Design review of the part built by this model. Coordinates are the model's own, in mm. Face numbers are marked on the shaded views. A direction names the side the tool comes from. Coordinates: 2 decimals unless noted, no trailing zeros. Loops run counter-clockwise (first coordinate to the right, second up) from the corner with the lowest first, then second, coordinate; pieces in that order, holes last. Notation, with made-up numbers: (-18, 49) - (24, 49) arc R12 cw to (24, 72) - close; hole circle Ø7 at (25.5, -40). An arc over 180 degrees is marked (long way). Use one line per item in the form item = value. Start each with the question number.
(1) Tool access review of the marked faces 1 and 2: name each direction out of +Z, -Z, +X, -X, +Y, -Y from which nothing blocks a thin tool from reaching the whole face with its end or side.
(2) Add section C-C (z = 3.95). State the section outline as (x, y) points.
(3) Add section D-D (z = 0.6). State the section outline as (x, y) points.
(4) Add section A-A (y = 0). State the section outline as (x, z) points.
(5) For L1, parallel to Z at x = -0.25, y = -7.5; L2, parallel to Y at x = -0.25, z = 1.65; L3, parallel to Z at x = -4.5, y = 1, list the stretches that pass through material, from the lowest coordinate up.
(6) Clearance check with a flat-ended pin moving along its axis: pin 1 Ø1 at (y, z) = (5, 1) entering from -X. State where the tip first meets the part, or that it passes through.
```python
from build123d import *

# Parameters (mm, degrees)
F0_R     = 11.5
F0_R_2   = 6.5
F1_DEPTH = 1.5
F0_R_3   = 4
F2_DEPTH = 2.5
F3_DEPTH = 5.5
F4_SIZE  = 1


with BuildPart() as f1:
    # F0 (on Top) → F1 (new body)
    with BuildSketch(Plane.XY):
        Circle(F0_R)
        Circle(F0_R_2, mode=Mode.SUBTRACT)
    extrude(amount=F1_DEPTH)

    # F0 (on Top) → F2 (join)
    with BuildSketch(Plane.XY):
        Circle(F0_R_2)
        Circle(F0_R_3, mode=Mode.SUBTRACT)
    extrude(amount=F2_DEPTH)

    # F0 (on Top) → F3 (join)
    with BuildSketch(Plane.XY):
        Circle(F0_R_3)
    extrude(amount=F3_DEPTH)

    # F4
    f4_edges = [f1.edges().sort_by_distance(p)[0] for p in [
        (-11.5, 0, 0),
    ]]
    chamfer(f4_edges, length=F4_SIZE)


solid = f1.part
```
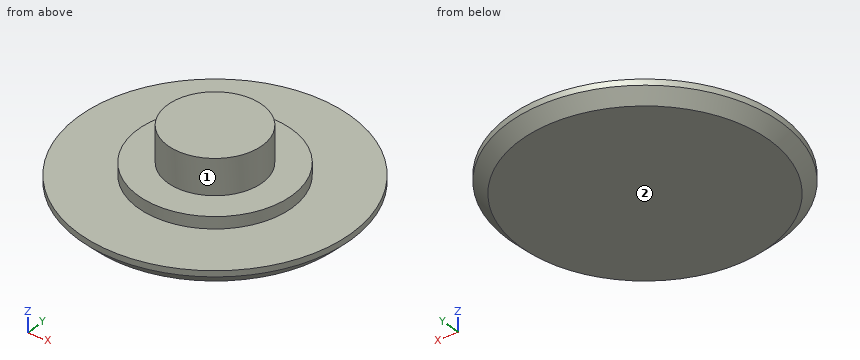
Computed values:
q1.face_1 = +Z
q1.face_2 = -Z, +X, -X, +Y, -Y
q2.outline = circle Ø8 at (0, 0)
q3.outline = circle Ø22.2 at (0, 0)
q4.outline = (-11.5, 1) - (-10.5, 0) - (10.5, 0) - (11.5, 1) - (11.5, 1.5) - (6.5, 1.5) - (6.5, 2.5) - (4, 2.5) - (4, 5.5) - (-4, 5.5) - (-4, 2.5) - (-6.5, 2.5) - (-6.5, 1.5) - (-11.5, 1.5) - close
q5.L1 = 0 to 1.5
q5.L2 = -6.5 to 6.5
q5.L3 = 0 to 2.5
q6.pin_1 = -10.58
